Study the drawing (mm; zero at the part's minimum x, y, z) and answer. A direction names the side the tool comes from. Coordinates: 2 decimals unless noted, no trailing zeros. Loops run counter-clockwise (first coordinate to the right, second up) from the corner with the lowest first, then second, coordinate; pieces in that order, holes last. Notation, with made-up numbers: (17, 39) -> (67, 39) arc R21 cw to (67, 61) -> close; hole circle Ø5 at (23, 74). An arc over 180 degrees is marked (long way). Answer in a Markdown table with one row per item.
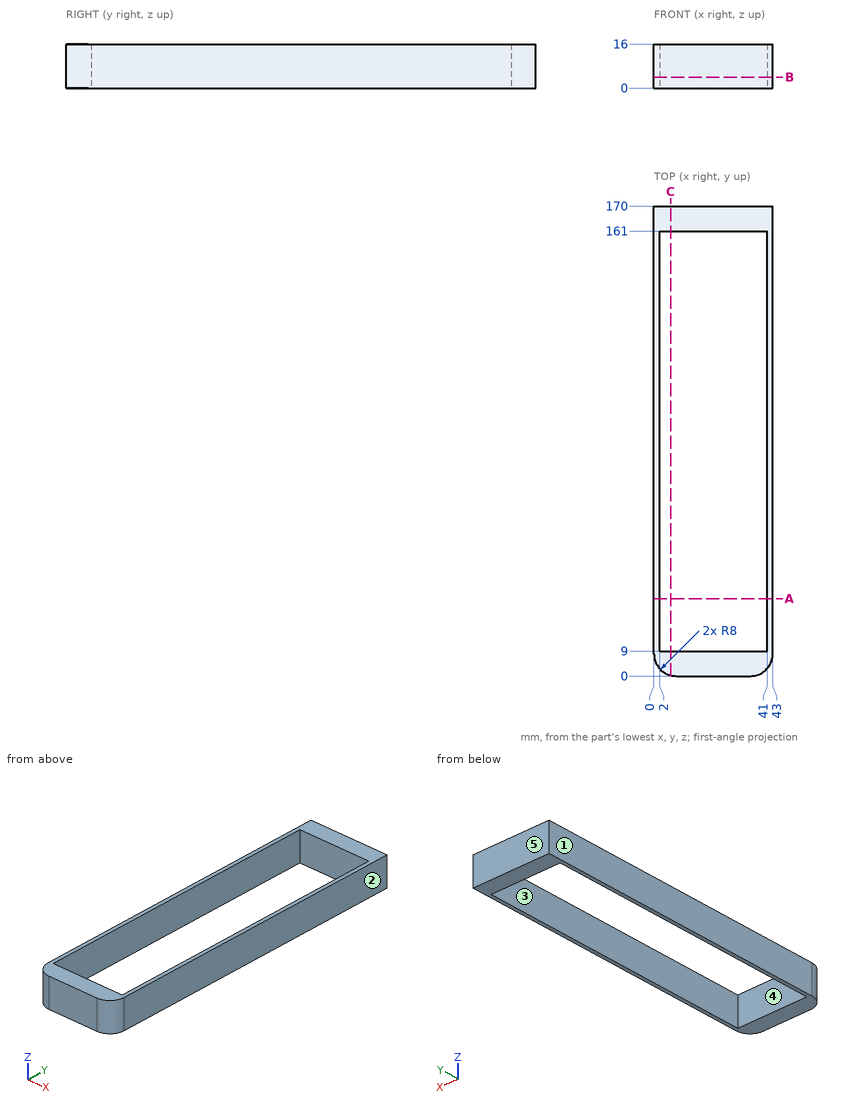
1. A cutting plane is placed at A-A on y = 28. Give the vertices of the cut face in (x, z), and give its area (3 significant figures).
A:
| item | result |
|---|---|
| outline | (0, 0) -> (2, 0) -> (2, 16) -> (0, 16) -> close; (41, 0) -> (43, 0) -> (43, 16) -> (41, 16) -> close |
| area | 64.0 mm2 |
2. A tool of negligible diameter and unlimited length cuts with its end or side. For the marked faces 4 and 5, from which of +Z, -Z, +X, -X, +Y, -Y can it reach the whole face along a straight path? Write none if from no direction.
A:
| item | result |
|---|---|
| face 4 | +Z, -Z |
| face 5 | +Z, -Z, +X, -X, +Y |
3. A cutting plane is placed at C-C on x = 6. Give the vertices of the cut face in (y, z), and give its area (3 significant figures).
A:
| item | result |
|---|---|
| outline | (0.25, 0) -> (9, 0) -> (9, 16) -> (0.25, 16) -> close; (161, 0) -> (170, 0) -> (170, 16) -> (161, 16) -> close |
| area | 284 mm2 |
4. Find the intervals of material crossed by probe 1 along X at (y, z) = (130, 14); probe 2 along Y at (x, z) = (21, 15); probe 3 along Y at (x, z) = (5, 11.75), in increasing order.
A:
| item | result |
|---|---|
| probe 1 | x = 0 to 2, 41 to 43 |
| probe 2 | y = 0 to 9, 161 to 170 |
| probe 3 | y = 0.58 to 9, 161 to 170 |
5. A cutting plane is placed at B-B on z = 4. Give the vertices of the cut face in (x, y).
A:
| item | result |
|---|---|
| outline | (0, 8) arc R8 ccw to (8, 0) -> (35, 0) arc R8 ccw to (43, 8) -> (43, 170) -> (0, 170) -> close; hole (2, 9) -> (41, 9) -> (41, 161) -> (2, 161) -> close |
6. The mould has two halves that part along X. Classify the marked faces 1, 2 and 3: pulls with the +X half, pulls with the -X half, needs draft (parallel to the pull), parting line crosses it, or undercut.
A:
| item | result |
|---|---|
| face 1 | pulls with the -X half |
| face 2 | pulls with the +X half |
| face 3 | undercut |
7. Given pin 1 Ø1.5 at (x, z) = (12.5, 5) entering from -Y, flat-ended and moving along its own axis, determine where the tip first touches the part or whether it passes through.
A:
| item | result |
|---|---|
| pin 1 | stops at y = 0 |
